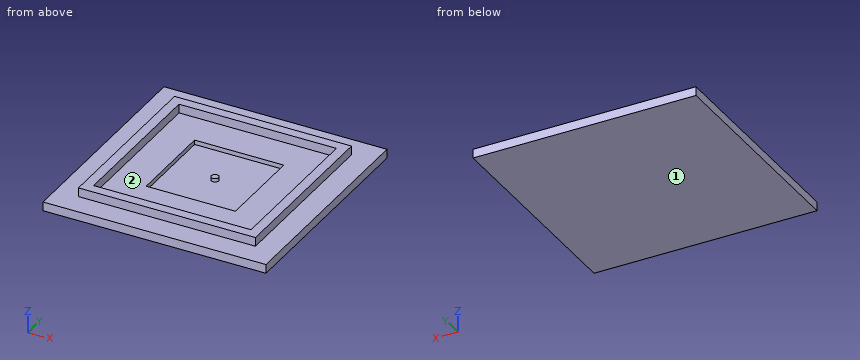
```python
from build123d import *

# Parameters (mm, degrees)
SKETCH1_W            = 127
SKETCH1_H            = 127
BOSS_EXTRUDE1_DEPTH  = 5.08
SKETCH2_W            = 100.838
SKETCH2_H            = 100.838
BOSS_EXTRUDE2_DEPTH  = 5.08
SKETCH3_W            = 89.662
SKETCH3_H            = 89.662
CUT_EXTRUDE1_DEPTH   = 5.08
SKETCH8_W            = 50.8
SKETCH8_H            = 50.8
CUT_EXTRUDE2_DEPTH   = 2.54
SKETCH9_R            = 2.032
BOSS_EXTRUDE10_DEPTH = 2.032


with BuildPart() as part:
    # Sketch1 → Boss-Extrude1 (new body)
    with BuildSketch(Plane.XY):
        Rectangle(SKETCH1_W, SKETCH1_H)
    extrude(amount=-BOSS_EXTRUDE1_DEPTH)

    # Sketch2 → Boss-Extrude2 (add)
    with BuildSketch(Plane.XY):
        Rectangle(SKETCH2_W, SKETCH2_H)
    extrude(amount=BOSS_EXTRUDE2_DEPTH)

    # Sketch3 → Cut-Extrude1 (cut)
    with BuildSketch(Plane.XY.offset(5.08)):
        Rectangle(SKETCH3_W, SKETCH3_H)
    extrude(amount=-CUT_EXTRUDE1_DEPTH, mode=Mode.SUBTRACT)

    # Sketch8 → Cut-Extrude2 (cut)
    with BuildSketch(Plane.XY):
        Rectangle(SKETCH8_W, SKETCH8_H)
    extrude(amount=-CUT_EXTRUDE2_DEPTH, mode=Mode.SUBTRACT)

    # Sketch9 → Boss-Extrude10 (add)
    with BuildSketch(Plane.XY.offset(-2.54)):
        Circle(SKETCH9_R)
    extrude(amount=BOSS_EXTRUDE10_DEPTH)


solid = part.part
```
Design review of the part built by this model. Coordinates are the model's own, in mm. Face numbers are marked on the shaded views. Round coordinates to 2 decimals unless told otherwise and drop trailing zeros. Order: outer loops, then holes, each group sorted by start corner. A loop starts at its lowest first (then second) coordinate and runs counter-clockwise, first axis right, second up. Notation, with made-up numbers: M -5,-17 L 31,-17 A12 ccw 31,-11 Z; hole C 36.25,72 d11. An arc over 180 degrees is marked long. Put each result on its own line as item: value.
Q1. Consider section C-C (y = 21). State the section outline as (x, z) points, and give its area (3 significant figures).
Reported:
outline: M -63.5,-5.08 L 63.5,-5.08 L 63.5,0 L 50.42,0 L 50.42,5.08 L 44.83,5.08 L 44.83,0 L 25.4,0 L 25.4,-2.54 L -25.4,-2.54 L -25.4,0 L -44.83,0 L -44.83,5.08 L -50.42,5.08 L -50.42,0 L -63.5,0 Z
area: 573 mm²
Q2. To check wall thickness, follow line 1 (X direction, y = 35, z = 4.5); line 2 (X direction, y = 15, z = -1.5). State the ranges of each line that lie inside material, in increasing order.
Reported:
line 1: -50.42 to -44.83, 44.83 to 50.42
line 2: -63.5 to -25.4, 25.4 to 63.5
Q3. Draft analysis for pull direction X (two halves, no side actions). For the marked faces 1 and 2, state which applies: released by +X, released by -X, zero draft, split by the parting line, or undercut.
Reported:
face 1: zero draft
face 2: undercut
Q4. Consider section A-A (x = 0). State the section outline as (y, z) points, and give its area (3 significant figures).
Reported:
outline: M -63.5,-5.08 L 63.5,-5.08 L 63.5,0 L 50.42,0 L 50.42,5.08 L 44.83,5.08 L 44.83,0 L 25.4,0 L 25.4,-2.54 L 2.03,-2.54 L 2.03,-0.51 L -2.03,-0.51 L -2.03,-2.54 L -25.4,-2.54 L -25.4,0 L -44.83,0 L -44.83,5.08 L -50.42,5.08 L -50.42,0 L -63.5,0 Z
area: 581 mm²
Q5. Consider section B-B (y = -43). State the section outline as (x, z) points.
Reported:
outline: M -63.5,-5.08 L 63.5,-5.08 L 63.5,0 L 50.42,0 L 50.42,5.08 L 44.83,5.08 L 44.83,0 L -44.83,0 L -44.83,5.08 L -50.42,5.08 L -50.42,0 L -63.5,0 Z
Q6. Insertion check: pin 1 Ø5.5 at (x, z) = (-21, 3.5) entering from +Y; pin 2 Ø10 at (x, y) = (-5.5, 25.5) entering from +Z; pin 3 Ø4 at (y, z) = (16.5, 3.5) entering from +X. Each pin has a flat end and moves straight along its axis. Give the tip position at first contact, or say it passes through.
Reported:
pin 1: y = 50.42
pin 2: z = 0
pin 3: x = 50.42
